Geometry: final body of the model. Coordinates: model frame, mm. A direction names the side the tool comes from. Give positions to 0.01 mm unless a question says otherwise; leave off trailing zeros. Write each loop counter-clockwise with the first axis right and the second up, starting at its lowest first coordinate (ties: lowest second). Pieces come first, ordered by that corner, then holes.
Q1. Pin query (flat end, axial travel): pin 1 (1.6 mm diameter, centred on y = 0, z = 0, fed in from -X). Return the tip coordinate at first contact, or that it passes through.
Q2. Line query: L1, parallel to X at y = -1.5, z = 1.2; L2, parallel to X at y = -1.25, z = -2.55; L3, parallel to Z at x = -65, y = 1.5. Output: solid intervals per line, ascending.
Q3. Draft query along Y for faces 4 (the face through (71.82, -0.24, -2.01)), 5 (the face through (-1, 0, -3)), 6 (the face through (-69.206, 0.4, 2.014)), 7 (the face through (-1, -5.351, 0)). Return one class per face: pulls with the +Y half, pulls with the -Y half, needs draft (parallel to the pull), parting line crosses it, or undercut.
Q4. Cut plane A-A on z = -1.9. Return the cut outline in (x, y), plus the area to 3 significant figures.
Q5. Reachability of faces 1 (the face through (-64, 0, -1)), 2 (the face through (64, 0, 1)), 3 (the face through (-69.206, 0.4, -2.014)) from +Z, -Z, +X, -X, +Y, -Y: full face, straight path, thin tool, end or side. Return the list, or none.
```python
from build123d import *

# Parameters (mm, degrees)
SKETCH19_W               = 115
SKETCH19_H               = 10
BOSS_EXTRUDE4_DEPTH      = 3
SKETCH21_R               = 2.5
BOSS_EXTRUDE13_DEPTH     = 2
MIRROR15_COPY_1_SKETCH_W = 115
MIRROR15_COPY_1_SKETCH_H = 10
MIRROR15_COPY_1_DEPTH    = 3
MIRROR15_COPY_2_SKETCH_R = 2.5
MIRROR15_COPY_2_DEPTH    = 2


with BuildPart() as part:
    # Sketch19 → Boss-Extrude4 (new body, symmetric)
    with BuildSketch(Plane.XY):
        with Locations((-0.678145843, -0.350765091)):
            Rectangle(SKETCH19_W, SKETCH19_H)
    boss_extrude4 = extrude(amount=BOSS_EXTRUDE4_DEPTH, both=True)

    # Sketch21 → Boss-Extrude13 (add)
    with BuildSketch(Plane.XY.offset(3)):
        with BuildLine():
            ThreePointArc((66.821854157, 4.649234909), (71.821854157, -0.350765091), (66.821854157, -5.350765091))
            Line((66.821854157, -5.350765091), (56.821854157, -5.350765091))
            Line((56.821854157, -5.350765091), (56.821854157, 4.649234909))
            Line((56.821854157, 4.649234909), (66.821854157, 4.649234909))
        make_face()
        with Locations((66.821854157, -0.350765091)):
            Circle(SKETCH21_R, mode=Mode.SUBTRACT)
    boss_extrude13 = extrude(amount=-BOSS_EXTRUDE13_DEPTH)

    # Mirror14: Boss-Extrude4, Boss-Extrude13 across plane
    add(boss_extrude4.mirror(Plane.XY))
    add(boss_extrude13.mirror(Plane.XY))

    # Mirror15: Boss-Extrude4, Boss-Extrude13 across plane
    add(boss_extrude4.mirror(Plane(origin=(0, 0, 0), x_dir=(0, 0, 1), z_dir=(1, 0, 0))))
    add(boss_extrude13.mirror(Plane(origin=(0, 0, 0), x_dir=(0, 0, 1), z_dir=(1, 0, 0))))

    # Mirror15 copy 1 sketch → Mirror15 copy 1 (add, symmetric)
    with BuildSketch(Plane(origin=(0, 0, 0), x_dir=(-1, 0, 0), z_dir=(0, 0, -1))):
        with Locations((-0.678145843, -0.350765091)):
            Rectangle(MIRROR15_COPY_1_SKETCH_W, MIRROR15_COPY_1_SKETCH_H)
    extrude(amount=MIRROR15_COPY_1_DEPTH, both=True)

    # Mirror15 copy 2 sketch → Mirror15 copy 2 (add)
    with BuildSketch(Plane(origin=(0, 0, -3), x_dir=(-1, 0, 0), z_dir=(0, 0, -1))):
        with BuildLine():
            ThreePointArc((66.821854157, 4.649234909), (71.821854157, -0.350765091), (66.821854157, -5.350765091))
            Line((66.821854157, -5.350765091), (56.821854157, -5.350765091))
            Line((56.821854157, -5.350765091), (56.821854157, 4.649234909))
            Line((56.821854157, 4.649234909), (66.821854157, 4.649234909))
        make_face()
        with Locations((66.821854157, -0.350765091)):
            Circle(MIRROR15_COPY_2_SKETCH_R, mode=Mode.SUBTRACT)
    extrude(amount=-MIRROR15_COPY_2_DEPTH)


solid = part.part
```
Data:
1. pin 1: stops at x = -58.18
2. L1: x = -71.69 to -69.04, -64.6 to 64.6, 69.04 to 71.69
2. L2: x = -71.74 to -69.15, -64.49 to 64.49, 69.15 to 71.74
2. L3: z = -3 to -1, 1 to 3
3. face 4: parting line crosses it
3. face 5: needs draft
3. face 6: undercut
3. face 7: pulls with the -Y half
4. outline: (-66.82, -5.35) - (66.82, -5.35) arc R5 ccw to (66.82, 4.65) - (-66.82, 4.65) arc R5 ccw to start; hole circle Ø5 at (-66.82, -0.35); hole circle Ø5 at (66.82, -0.35)
4. area: 1,380 mm2
5. face 1: -X, +Y, -Y
5. face 2: +X, +Y, -Y
5. face 3: +Z, -Z
